from build123d import *
from OCP.BRepFilletAPI import BRepFilletAPI_MakeChamfer

# Parameters (mm, degrees)
BOSS_EXTRUDE1_DEPTH = 10.25
BOSS_EXTRUDE2_DEPTH = 1
BOSS_EXTRUDE3_DEPTH = 1
FILLET1_R           = 1
CHAMFER1_SIZE       = 0.25
CHAMFER1_SIZE2      = 0.175051885


with BuildPart() as part:
    # Sketch1 → Boss-Extrude1 (new, symmetric)
    with BuildSketch(Plane(origin=(0, 0, 0), x_dir=(1, 0, 0), z_dir=(0, 1, 0))):
        with BuildLine():
            Line((5.5, 5.099019514), (5.5, -5.099019514))
            ThreePointArc((5.5, -5.099019514), (-7.5, 0), (5.5, 5.099019514))
        make_face()
    extrude(amount=BOSS_EXTRUDE1_DEPTH, both=True)

    # Sketch2 → Boss-Extrude2 (add, symmetric)
    with BuildSketch(Plane(origin=(0, 6.5, 0), x_dir=(1, 0, 0), z_dir=(0, 1, 0))):
        with BuildLine():
            Line((6, 5.291502622), (6, -5.291502622))
            ThreePointArc((6, -5.291502622), (-8, 0), (6, 5.291502622))
        make_face()
    extrude(amount=BOSS_EXTRUDE2_DEPTH, both=True)

    # Sketch3 → Boss-Extrude3 (add, symmetric)
    with BuildSketch(Plane(origin=(0, -6.5, 0), x_dir=(1, 0, 0), z_dir=(0, 1, 0))):
        with BuildLine():
            Line((6, -5.291502622), (6, 5.291502622))
            ThreePointArc((6, 5.291502622), (-8, 0), (6, -5.291502622))
        make_face()
    extrude(amount=BOSS_EXTRUDE3_DEPTH, both=True)

    # Fillet1
    # the kernel refuses this fillet: 1 mm, written as the material it takes off along each edge
    with BuildSketch(Plane(origin=(0, 7.5, 0), x_dir=(0.8999821902414007, 0, 0.43592666498883875), z_dir=(0.43592666498883875, 0, -0.8999821902414007))) as fillet1_piece_1:
        with BuildLine():
            CenterArc((7, 0.866025404), FILLET1_R, 300, 60)
            Line((7.5, 0), (7.51, -0.017320508))
            ThreePointArc((7.51, -0.017320508), (7.75, -0.02), (8, -0.02))
            Line((8, -0.02), (8.02, 0))
            Line((8.02, 0), (8.02, 0.866025404))
            Line((8.02, 0.866025404), (8, 0.866025404))
        make_face()
    revolve(axis=Axis((0, 7.5, 0), (0, -1, 0)), revolution_arc=308.311452645, mode=Mode.SUBTRACT)
    with BuildSketch(Plane(origin=(6, 7.5, -7.456566132), x_dir=(0, -1, 0), z_dir=(0, 0, 1))) as fillet1_piece_2:
        with BuildLine():
            CenterArc((0.866025404, -1), FILLET1_R, 90, 60)
            Line((0, -0.5), (-0.017320508, -0.49))
            ThreePointArc((-0.017320508, -0.49), (-0.02, -0.25), (-0.02, 0))
            Line((-0.02, 0), (0, 0.02))
            Line((0, 0.02), (0.866025404, 0.02))
            Line((0.866025404, 0.02), (0.866025404, 0))
        make_face()
    extrude(amount=14.913132263, mode=Mode.SUBTRACT)
    with BuildSketch(Plane(origin=(6, -7.5, 7.456566132), x_dir=(-1, 0, 0), z_dir=(0, 0, -1))) as fillet1_piece_3:
        with BuildLine():
            CenterArc((1, 0.866025404), FILLET1_R, 180, 60)
            Line((0, 0.866025404), (-0.02, 0.866025404))
            Line((-0.02, 0.866025404), (-0.02, 0))
            Line((-0.02, 0), (0, -0.02))
            ThreePointArc((0, -0.02), (0.25, -0.02), (0.49, -0.017320508))
            Line((0.49, -0.017320508), (0.5, 0))
        make_face()
    extrude(amount=14.913132263, mode=Mode.SUBTRACT)
    with BuildSketch(Plane(origin=(0, -7.5, 0), x_dir=(0.8999821902414012, 0, -0.4359266649888379), z_dir=(0.4359266649888379, 0, 0.8999821902414012))) as fillet1_piece_4:
        with BuildLine():
            CenterArc((7, 0.866025404), FILLET1_R, 300, 60)
            Line((8, 0.866025404), (8.02, 0.866025404))
            Line((8.02, 0.866025404), (8.02, 0))
            Line((8.02, 0), (8, -0.02))
            ThreePointArc((8, -0.02), (7.75, -0.02), (7.51, -0.017320508))
            Line((7.51, -0.017320508), (7.5, 0))
        make_face()
    revolve(axis=Axis((0, -7.5, 0), (0, 1, 0)), revolution_arc=308.311452645, mode=Mode.SUBTRACT)

    # Chamfer1: one chamfer whose edges measure the first distance from different faces: ONE call of the kernel's chamfer builder (chamfer() names one face for all edges)
    chamfer1_edges_1 = [part.edges().sort_by_distance(p)[0] for p in [
        (-8, 5.5, 0),
        (6, 5.5, 0),
    ]]
    chamfer1_side_1 = [part.faces().sort_by_distance(p)[0] for p in [
        (5.787397084, 5.5, 0),
    ]]
    chamfer1_edges_2 = [part.edges().sort_by_distance(p)[0] for p in [
        (6, -5.5, 0),
    ]]
    chamfer1_side_2 = [part.faces().sort_by_distance(p)[0] for p in [
        (6, -6.066987298, 0),
    ]]
    chamfer1_edges_3 = [part.edges().sort_by_distance(p)[0] for p in [
        (-8, -5.5, 0),
    ]]
    chamfer1_side_3 = [part.faces().sort_by_distance(p)[0] for p in [
        (-8, -6.066987298, 0),
    ]]
    chamfer1 = BRepFilletAPI_MakeChamfer(part.part.solid().wrapped)
    for e in chamfer1_edges_1:
        chamfer1.Add(CHAMFER1_SIZE, CHAMFER1_SIZE2, e.wrapped, chamfer1_side_1[0].wrapped)  # the first distance lies on this face
    for e in chamfer1_edges_2:
        chamfer1.Add(CHAMFER1_SIZE, CHAMFER1_SIZE2, e.wrapped, chamfer1_side_2[0].wrapped)  # the first distance lies on this face
    for e in chamfer1_edges_3:
        chamfer1.Add(CHAMFER1_SIZE, CHAMFER1_SIZE2, e.wrapped, chamfer1_side_3[0].wrapped)  # the first distance lies on this face
    add(Compound.cast(chamfer1.Shape()), mode=Mode.REPLACE)


solid = part.part
Verification items for the finished model (mm, model axes). A direction names the side the tool comes from. Coordinates: 2 decimals unless noted, no trailing zeros. Loops run counter-clockwise (first coordinate to the right, second up) from the corner with the lowest first, then second, coordinate; pieces in that order, holes last. Notation, with made-up numbers: M 71,54.25 L 85,54.25 A29 cw 85,74.25 Z; hole C 31.5,15 d3. An arc over 180 degrees is marked long. One line per item, written item: value.
1. Section check C-C on y = -8. Record the cut outline in (x, z), plus the area to 3 significant figures.
Answers follow:
outline: M 5.5,-5.1 L 5.5,5.1 A7.5 ccw long Z
area: 163 mm^2
2. Set-up check for faces 1 (the cylindrical face through (-7.496, 8.894, 0.251)), 2 (the cylindrical face through (-7.496, -8.856, 0.251)), 3 (the flat face through (5.5, 9, 0)), 4 (the cylindrical face through (-7.496, 0.077, 0.251)): record each of +Z, -Z, +X, -X, +Y, -Y from which the full face is reachable in a straight line by a thin tool's end or side.
Answers follow:
face 1: +Y
face 2: -Y
face 3: +Z, -Z, +X, +Y
face 4: none
3. Section check B-B on x = 0. Record the cut outline in (y, z).
Answers follow:
outline: M -10.25,-7.5 L -7.5,-7.5 A1 ccw -6.63,-8 L -5.75,-8 L -5.5,-7.82 L -5.5,-7.5 L 5.5,-7.5 L 5.5,-7.75 L 5.68,-8 L 6.63,-8 A1 ccw 7.5,-7.5 L 10.25,-7.5 L 10.25,7.5 L 7.5,7.5 A1 ccw 6.63,8 L 5.68,8 L 5.5,7.75 L 5.5,7.5 L -5.5,7.5 L -5.5,7.82 L -5.75,8 L -6.63,8 A1 ccw -7.5,7.5 L -10.25,7.5 Z
4. Mould release check, pull along Y, two halves, no side actions. Record for faces 5 (the cylindrical face through (-8, 6, 0)), 6 (the flat face through (-1, 10.25, 0)), 7 (the conical face through (-7.872, 5.589, 0.267)): pulls with the +Y half, pulls with the -Y half, needs draft (parallel to the pull), parting line crosses it, or undercut.
Answers follow:
face 5: needs draft
face 6: pulls with the +Y half
face 7: undercut
5. Section check A-A on z = 0. Record the cut outline in (x, y), plus the area to 3 significant figures.
Answers follow:
outline: M -8,-6.63 A1 ccw -7.5,-7.5 L -7.5,-10.25 L 5.5,-10.25 L 5.5,-7.5 A1 ccw 6,-6.63 L 6,-5.75 L 5.82,-5.5 L 5.5,-5.5 L 5.5,5.5 L 5.75,5.5 L 6,5.68 L 6,6.63 A1 ccw 5.5,7.5 L 5.5,10.25 L -7.5,10.25 L -7.5,7.5 A1 ccw -8,6.63 L -8,5.68 L -7.75,5.5 L -7.5,5.5 L -7.5,-5.5 L -7.82,-5.5 L -8,-5.75 Z
area: 270 mm^2
6. Material ranges on line 1 along X through (y, z) = (-4, 5.5); line 2 along Z through (x, y) = (4.5, 2.5); line 3 along Z through (x, y) = (-3, 6.75), recorded low to high. Write a range as from..to.
Answers follow:
line 1: -5.1..5.1
line 2: -6..6
line 3: -7.41..7.41
7. Gauge pin test, flat ends, axial feed: P1, Ø5, axis at x = -5.5, y = 3.5, coming from the -Z side; P2, Ø1.5, axis at y = 2.5, z = -4, coming from the -X side; P3, Ø4, axis at y = -6, z = -3, coming from the -X side. Record the tip position at first contact, or that the pin passes through.
Answers follow:
P1: z = -6.87
P2: x = -6.76
P3: x = -7.94
